Can you work these out from the model? Positions are in its coordinate system, mm. A direction names the side the tool comes from. Round coordinates to 2 decimals unless told otherwise and drop trailing zeros. Loops run counter-clockwise (first coordinate to the right, second up) from the corner with the lowest first, then second, coordinate; pieces in that order, holes last. Notation, with made-up numbers: (20.25, 86.25) -> (67.25, 86.25) arc R21 cw to (67.25, 91.25) -> close; hole circle Ø10 at (-31, -4.75). An arc over 180 degrees is marked (long way). Use a Markdown table: item, result.
Autodesk Inventor part; units mm, degrees
ref_plane "Work Plane1" through (20, 14.5, 0) normal (1, 0, 0) x (0, 1, 0)
ref_plane "Work Plane2" through (0, 14.5, -20) normal (0, 0, -1) x (-1, 0, 0)
ref_plane "YZ Plane" through (0, 0, 0) normal (1, 0, 0) x (0, 1, 0)
sketch "Sketch1" plane through (0, 0, 0) normal (0, 1, 0) x (-1, 0, 0)
  circle A0 centre (0, 0) radius 20
  dimension "d0" = 40
extrude "Extrusion1" add sketch "Sketch1" along normal blind 10
sketch "Sketch2" plane through (0, 10, 0) normal (0, 1, 0) x (1, 0, 0)
  circle A0 centre (0, 0) radius 17.5
  circle A1 centre (0, 0) radius 20
  line L0 (-18.3303, 8) -> (-15.5644, 8)
  line L1 (-18.3303, -8) -> (-15.5644, -8)
  circle A2 centre (0, 0) radius 20
  point P0 (-16.9473, 8)
  dimension "d3" = 35
  dimension "d4" = 8
  dimension "d5" = 8
  dimension "d6" = 40
extrude "Extrusion2" add sketch "Sketch2" along normal blind 4.5 contours A0 L0 A1 L1 picked at (18.7918, -3.0381)
sketch "Sketch3" plane through (0, 10, 0) normal (0, 1, 0) x (1, 0, 0)
  circle A0 centre (0, 0) radius 17.5
extrude "Extrusion3" cut sketch "Sketch3" against normal blind 8
sketch "Sketch4" plane through (0, 14.5, 0) normal (0, 1, 0) x (1, 0, 0)
  circle A0 centre (0, 0) radius 20
  point P0 (0, -20.0355)
  point P1 (20, 0)
  point P2 (0, 20)
ref_plane "Work Plane1" through (20, 14.5, 0) normal (1, 0, 0) x (0, 1, 0)
sketch "Sketch5" plane through (20, 14.5, 0) normal (1, 0, 0) x (0, 1, 0)
  circle A0 centre (-2.5, 0) radius 1.6
  line L0 (0, -20) -> (0, 20)
  point P0 (-14.5, 0)
  point P1 (0, 8)
  point P2 (0, -8)
  dimension "d11" = 3.2
  dimension "d12" = 2.5
extrude "Extrusion4" cut sketch "Sketch5" against normal up to surface
ref_plane "Work Plane2" through (0, 14.5, -20) normal (0, 0, -1) x (-1, 0, 0)
sketch "Sketch6" plane through (0, 14.5, -20) normal (0, 0, -1) x (-1, 0, 0)
  circle A0 centre (0, -2.5) radius 1.6
  line L0 (18.3303, 0) -> (-20, 0)
  point P0 (0, -14.5)
  dimension "d15" = 3.2
  dimension "d16" = 2.5
extrude "Extrusion5" cut sketch "Sketch6" against normal through all
sketch "Sketch7" plane through (0, 10, 0) normal (0, 1, 0) x (1, 0, 0)
  line L0 (-13, -3.3) -> (-13, 5.1)
  line L1 (-13, 5.1) -> (-18.25, 5.1)
  line L2 (-18.25, 5.1) -> (-18.25, -3.3)
  line L3 (-16.25, -5.3) -> (-15, -5.3)
  arc A0 (-15, -5.3) -> (-13, -3.3) centre (-15, -3.3) ccw
  arc A1 (-18.25, -3.3) -> (-16.25, -5.3) centre (-16.25, -3.3) ccw
  arc A2 (-18.3303, 8) -> (-18.3303, -8) centre (0, 0) ccw
  point P0 (-18.25, -5.3)
  dimension "d19" = 10.4
  dimension "d20" = 5.25
  dimension "d21" = 2
  dimension "d25" = 18.25
  dimension "d26" = 5.1
extrude "Extrusion6" [suppressed]
properties part number "Payload Adapter V2 No XT30"
1. I want a section at D-D (x = -10.5). Please give me the cut outline in (y, z).
Answer sheet:
| item | result |
|---|---|
| outline | (0, -17.02) -> (14.5, -17.02) -> (14.5, -14) -> (2, -14) -> (2, 14) -> (14.5, 14) -> (14.5, 17.02) -> (0, 17.02) -> close |
2. Will these pins go through, and if not, where does the flat tip stop? pin 1 Ø4 at (x, z) = (6, 10) entering from +Y; pin 2 Ø5 at (x, y) = (-4.5, 9) entering from +Z; pin 3 Ø6 at (y, z) = (6, -11) entering from +X.
Answer sheet:
| item | result |
|---|---|
| pin 1 | stops at y = 2 |
| pin 2 | stops at z = 19.9 |
| pin 3 | stops at x = 18.33 |
3. I need wall thicknesses on line 1 (Z direction, x = 0, y = 3.5); line 2 (Y direction, x = 18.7, z = 0); line 3 (Z direction, x = -3.5, y = 4.5). Which ranges of each line are inside material? Lowest first, please.
Answer sheet:
| item | result |
|---|---|
| line 1 | z = -20 to -17.5, 17.5 to 20 |
| line 2 | y = 0 to 10.4, 13.6 to 14.5 |
| line 3 | z = -19.69 to -17.15, 17.15 to 19.69 |
4. I want a section at A-A (x = 0). Please give me the cut outline in (y, z), plus the area to 4 significant figures.
Answer sheet:
| item | result |
|---|---|
| outline | (0, -20) -> (10.4, -20) -> (10.4, -17.5) -> (2, -17.5) -> (2, 17.5) -> (10.4, 17.5) -> (10.4, 20) -> (0, 20) -> close; (13.6, -20) -> (14.5, -20) -> (14.5, -17.5) -> (13.6, -17.5) -> close; (13.6, 17.5) -> (14.5, 17.5) -> (14.5, 20) -> (13.6, 20) -> close |
| area | 126.5 mm² |
5. I want a section at B-B (z = 3.5). Please give me the cut outline in (x, y), plus the area to 3 significant figures.
Answer sheet:
| item | result |
|---|---|
| outline | (-19.69, 0) -> (19.69, 0) -> (19.69, 14.5) -> (17.15, 14.5) -> (17.15, 2) -> (-17.15, 2) -> (-17.15, 10) -> (-19.69, 10) -> close |
| area | 131 mm² |
6. Which directions (+Z, -Z, +X, -X, +Y, -Y) give clear straight access to the entire face, cutting with the end or side of a thin tool? Please do faces 1 (the flat face through (-18, 10, 0)), 2 (the flat face through (0, 2, 0)), 3 (the flat face through (0, 0, 0)).
Answer sheet:
| item | result |
|---|---|
| face 1 | -X, +Y |
| face 2 | +Y |
| face 3 | +Z, -Z, +X, -X, -Y |
7. I want a section at C-C (y = 12). Please give me the cut outline in (x, z), plus the area to 3 significant figures.
Answer sheet:
| item | result |
|---|---|
| outline | (-18.33, -8) arc R20 ccw to (-1.6, -19.94) -> (-1.6, -17.43) arc R17.5 cw to (-15.56, -8) -> close; (-18.33, 8) -> (-15.56, 8) arc R17.5 cw to (-1.6, 17.43) -> (-1.6, 19.94) arc R20 ccw to start; (1.6, -19.94) arc R20 ccw to (19.94, -1.6) -> (17.43, -1.6) arc R17.5 cw to (1.6, -17.43) -> close; (1.6, 17.43) arc R17.5 cw to (17.43, 1.6) -> (19.94, 1.6) arc R20 ccw to (1.6, 19.94) -> close |
| area | 229 mm² |
8. If we mould it in two halves opening along X, with no side actions, what happens to faces 4 (the cylindrical face through (0.208, 13.586, 18.695)), 5 (the flat face through (-17, 12, -8))? For each: +X half, -X half, draft (parallel to the pull), parting line (faces both ways), or undercut.
Answer sheet:
| item | result |
|---|---|
| face 4 | undercut |
| face 5 | draft |
